```python
from build123d import *

# Parameters (mm, degrees)
F0_R     = 25.4
F1_DEPTH = 152.4
F3_DEPTH = 304.801
F4_R     = 21.59
F5_DEPTH = 304.801


with BuildPart() as f1:
    # F0 (on Front) → F1 (new body, symmetric)
    with BuildSketch(Plane.XZ):
        Circle(F0_R)
    extrude(amount=F1_DEPTH, both=True)

    # F2 (on face) → F3 (cut, through all)
    with BuildSketch(Plane.XZ.offset(152.4)):
        with BuildLine():
            Line((0, 25.4), (0, 0))
            Line((0, 0), (25.4, 0))
            ThreePointArc((25.4, 0), (17.960512, 17.960512), (0, 25.4))
        make_face()
    extrude(amount=-F3_DEPTH, mode=Mode.SUBTRACT)

    # F4 (on face) → F5 (cut, through all)
    with BuildSketch(Plane.XZ.offset(152.4)):
        Circle(F4_R)
    extrude(amount=-F5_DEPTH, mode=Mode.SUBTRACT)


solid = f1.part
```
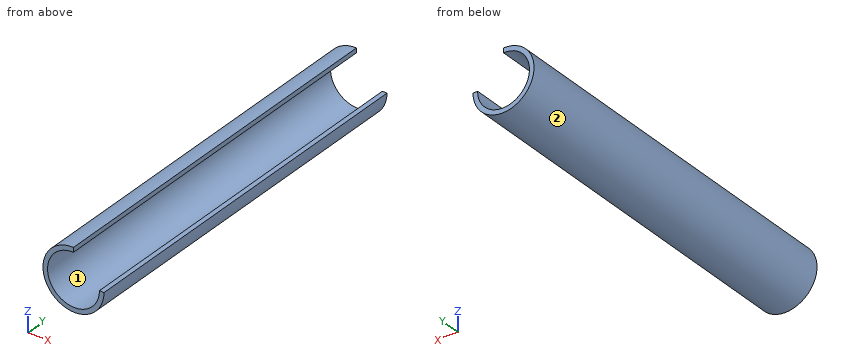
Geometry: final body of the model. Coordinates: model frame, mm. Face numbers are marked on the shaded views. Round coordinates to 2 decimals unless told otherwise and drop trailing zeros. Write each loop counter-clockwise with the first axis right and the second up, starting at its lowest first coordinate (ties: lowest second). Pieces come first, ordered by that corner, then holes. Notation, with made-up numbers: M -17.5,-9.5 L 11.5,-9.5 A21 cw 11.5,-2.5 Z; hole C 40,85 d4. An arc over 180 degrees is marked long. Answer in a Markdown table with one row per item. Add a question column.
(1) Cut plane C-C, the plane x = 7. Return the cut outline in (y, z), then the cut area to 3 significant figures.
(2) Ray query, L1, parallel to X at y = 0, z = -6; L2, parallel to X at y = 8, z = -13; L3, parallel to Z at x = -3.5, y = -1. Return the intervals inside material, ascending.
(3) Cut plane B-B, the plane y = -21. Return the cut outline in (x, z), then the cut area to 3 significant figures.
(4) Cut plane A-A, the plane z = -8. Return the cut outline in (x, y).
(5) Contact query for flat-ended pins moving along their axis: pin 1 (1 mm diameter, centred on x = 0.5, y = -31.5, fed in from -Z); pin 2 (3 mm diameter, centred on y = 68.5, z = 23.5, fed in from +X); pin 3 (2 mm diameter, centred on y = 86.5, z = -20, fed in from -X). Output: stop coordinate, or through.
(6) Draft query along Z for the marked faces 1 and 2. Return one class per face: pulls with the +Z half, pulls with the -Z half, needs draft (parallel to the pull), parting line crosses it, or undercut.
Established:
| question | item | result |
|---|---|---|
| 1 | outline | M -152.4,-24.42 L 152.4,-24.42 L 152.4,-20.42 L -152.4,-20.42 Z |
| 1 | area | 1,220 mm² |
| 2 | L1 | -24.68 to -20.74, 20.74 to 24.68 |
| 2 | L2 | -21.82 to -17.24, 17.24 to 21.82 |
| 2 | L3 | -25.16 to -21.3, 21.3 to 25.16 |
| 3 | outline | M 0,21.59 L 0,25.4 A25.4 ccw long 25.4,0 L 21.59,0 A21.59 cw long Z |
| 3 | area | 422 mm² |
| 4 | outline | M -24.11,-152.4 L -20.05,-152.4 L -20.05,152.4 L -24.11,152.4 Z; M 20.05,-152.4 L 24.11,-152.4 L 24.11,152.4 L 20.05,152.4 Z |
| 5 | pin 1 | z = -25.4 |
| 5 | pin 2 | x = 0 |
| 5 | pin 3 | x = -16.86 |
| 6 | face 1 | undercut |
| 6 | face 2 | parting line crosses it |
